from build123d import *

# Parameters (mm, degrees)
SKETCH_R        = 7.5
SKETCH_R_2      = 4.25
PAD_DEPTH       = 75
SKETCH001_W     = 19.415184
SKETCH001_H     = 42
POCKET_DEPTH    = 42
SKETCH002_R     = 11.25
POCKET001_DEPTH = 5
SKETCH003_R     = 1.75
HOLE_DEPTH      = 25
SKETCH004_R     = 1.5
HOLE001_DEPTH   = 25
HOLE001_TIPS_R  = 1.5
SKETCH005_R     = 11
POCKET002_DEPTH = 33
SKETCH006_R     = 11
POCKET003_DEPTH = 33


with BuildPart() as part:
    # Sketch → Pad (new body)
    with BuildSketch(Plane.XY):
        with BuildLine():
            ThreePointArc((-38.9, 12.5), (-51.4, 0), (-38.9, -12.5))
            Line((-38.9, -12.5), (30.9, -12.5))
            Line((95.9, -12.5), (30.9, -12.5))
            Line((95.9, -7.5), (95.9, -12.5))
            Line((34.678675, 11.915184), (95.9, -7.5))
            ThreePointArc((34.678675, 11.915184), (32.811831, 12.352931), (30.9, 12.5))
            Line((-38.9, 12.5), (30.9, 12.5))
        make_face()
        with Locations((-38.9, 0)):
            Circle(SKETCH_R, mode=Mode.SUBTRACT)
        with Locations((30.9, 0)):
            Circle(SKETCH_R_2, mode=Mode.SUBTRACT)
    extrude(amount=PAD_DEPTH)

    # Sketch001 (on Face3 of Pad) → Pocket (cut)
    with BuildSketch(Plane.YZ.offset(95.9)):
        with Locations((2.207592, 37.5)):
            Rectangle(SKETCH001_W, SKETCH001_H)
    extrude(amount=-POCKET_DEPTH, mode=Mode.SUBTRACT)

    # Sketch002 (on Face11 of Pocket) → Pocket001 (cut)
    with BuildSketch(Plane(origin=(0, -7.5, 0), x_dir=(-1, 0, 0), z_dir=(0, 1, 0))):
        with Locations((-74.9, 37.5)):
            Circle(SKETCH002_R)
    extrude(amount=-POCKET001_DEPTH, mode=Mode.SUBTRACT)

    # Sketch003 (on Face12 of Pocket001) → Hole (cut)
    with BuildSketch(Plane(origin=(0, -7.5, 0), x_dir=(-1, 0, 0), z_dir=(0, 1, 0))):
        with Locations((-90.4, 53)):
            Circle(SKETCH003_R)
        with Locations((-59.4, 53)):
            Circle(SKETCH003_R)
        with Locations((-59.4, 22)):
            Circle(SKETCH003_R)
        with Locations((-90.4, 22)):
            Circle(SKETCH003_R)
    extrude(amount=-HOLE_DEPTH, mode=Mode.SUBTRACT)

    # Sketch004 (on Face3 of Hole) → Hole001 (cut)
    with BuildSketch(Plane.XZ.offset(12.5)):
        with Locations((1.1, 72)):
            Circle(SKETCH004_R)
        with Locations((1.1, 54)):
            Circle(SKETCH004_R)
        with Locations((1.1, 21)):
            Circle(SKETCH004_R)
        with Locations((1.1, 3)):
            Circle(SKETCH004_R)
    extrude(amount=-HOLE001_DEPTH, mode=Mode.SUBTRACT)

    # Hole001 tips → Hole001 tip 1 section 0
    with BuildSketch(Plane.XZ.offset(-12.5), mode=Mode.PRIVATE) as hole001_tip_1_s0:
        with Locations((1.1, 72)):
            Circle(HOLE001_TIPS_R)
    loft([hole001_tip_1_s0.sketch, Vertex(1.1, 13.401291, 72)], mode=Mode.SUBTRACT)

    # Hole001 tips → Hole001 tip 2 section 0
    with BuildSketch(Plane.XZ.offset(-12.5), mode=Mode.PRIVATE) as hole001_tip_2_s0:
        with Locations((1.1, 54)):
            Circle(HOLE001_TIPS_R)
    loft([hole001_tip_2_s0.sketch, Vertex(1.1, 13.401291, 54)], mode=Mode.SUBTRACT)

    # Hole001 tips → Hole001 tip 3 section 0
    with BuildSketch(Plane.XZ.offset(-12.5), mode=Mode.PRIVATE) as hole001_tip_3_s0:
        with Locations((1.1, 21)):
            Circle(HOLE001_TIPS_R)
    loft([hole001_tip_3_s0.sketch, Vertex(1.1, 13.401291, 21)], mode=Mode.SUBTRACT)

    # Hole001 tips → Hole001 tip 4 section 0
    with BuildSketch(Plane.XZ.offset(-12.5), mode=Mode.PRIVATE) as hole001_tip_4_s0:
        with Locations((1.1, 3)):
            Circle(HOLE001_TIPS_R)
    loft([hole001_tip_4_s0.sketch, Vertex(1.1, 13.401291, 3)], mode=Mode.SUBTRACT)

    # Sketch005 (on Face5 of Hole001) → Pocket002 (cut)
    with BuildSketch(Plane.XY.offset(75)):
        with Locations((30.9, 0)):
            Circle(SKETCH005_R)
    extrude(amount=-POCKET002_DEPTH, mode=Mode.SUBTRACT)

    # Sketch006 (on Face4 of Pocket002) → Pocket003 (cut)
    with BuildSketch(Plane(origin=(0, 0, 0), x_dir=(1, 0, 0), z_dir=(0, 0, -1))):
        with Locations((30.9, 0)):
            Circle(SKETCH006_R)
    extrude(amount=-POCKET003_DEPTH, mode=Mode.SUBTRACT)


solid = part.part
The model under review builds one solid part; all positions refer to its coordinate system, in mm. A direction names the side the tool comes from. Round coordinates to 2 decimals unless told otherwise and drop trailing zeros. Loops run counter-clockwise (first coordinate to the right, second up) from the corner with the lowest first, then second, coordinate; pieces in that order, holes last. Notation, with made-up numbers: (75.25, 54) -> (85.25, 54) arc R4 cw to (85.25, 58) -> close; hole circle Ø7 at (-11.5, 48). An arc over 180 degrees is marked (long way). Return JSON: item names as keys, results as strings.
(1) For pin 1 (3 mm diameter, centred on x = 61.5, z = 60, fed in from +Y) (3 decimals); pin 2 (11 mm diameter, centred on x = 30.9, y = 0, fed in from -Z); pin 3 (2 mm diameter, centred on x = 59.5, z = 48.5, fed in from +Y), all flat-tipped, find the tip position at first contact; note any pin that passes through.
Solved:
{"pin 1": "y = 3.885", "pin 2": "z = 33", "pin 3": "y = -7.5"}
(2) For faces 4 (the flat face through (66, -7.5, 47)), 5 (the cylindrical face through (35.976, -9.759, 58.731)), 6 (the flat face through (31, 5, 33)), 7 (the flat face through (51.256, 6.658, 36.975)), list the 3-axis set-ups (+Z, -Z, +X, -X, +Y, -Y) from which the entire face can be reached by the end or side of a thin tool; tool diameter is ignored.
Solved:
{"face 4": "+X, +Y", "face 5": "+Z", "face 6": "-Z", "face 7": "+Z, -Z, +X, +Y"}
(3) Add section B-B on y = 0. Write out the cut boundary in (x, z), plus the area to 3 significant figures.
Solved:
{"outline": "(-51.4, 0) -> (-46.4, 0) -> (-46.4, 75) -> (-51.4, 75) -> close; (-31.4, 0) -> (19.9, 0) -> (19.9, 33) -> (26.65, 33) -> (26.65, 42) -> (19.9, 42) -> (19.9, 75) -> (-31.4, 75) -> close; (35.15, 33) -> (41.9, 33) -> (41.9, 0) -> (72.25, 0) -> (72.25, 16.5) -> (53.9, 16.5) -> (53.9, 58.5) -> (72.25, 58.5) -> (72.25, 75) -> (41.9, 75) -> (41.9, 42) -> (35.15, 42) -> close; hole circle Ø3 at (1.1, 3); hole circle Ø3 at (1.1, 21); hole circle Ø3 at (1.1, 54); hole circle Ø3 at (1.1, 72)", "area": "5,820 mm2"}
(4) For line 1 (Z direction, x = 90.4, y = -10.1); line 2 (Y direction, x = 30.9, z = 68.5); line 3 (Z direction, x = 1.1, y = -5.5), list the stretches that pass through material, from the lowest coordinate up.
Solved:
{"line 1": "0 to 20.25, 23.75 to 51.25, 54.75 to 75", "line 2": "-12.5 to -11, 11 to 12.5", "line 3": "0 to 1.5, 4.5 to 19.5, 22.5 to 52.5, 55.5 to 70.5, 73.5 to 75"}
(5) Add section C-C on x = 79. Write out the cut boundary in (y, z).
Solved:
{"outline": "(-12.5, 0) -> (-2.14, 0) -> (-2.14, 16.5) -> (-7.5, 16.5) -> (-7.5, 27.02) -> (-12.5, 27.02) -> close; (-12.5, 47.98) -> (-7.5, 47.98) -> (-7.5, 58.5) -> (-2.14, 58.5) -> (-2.14, 75) -> (-12.5, 75) -> close"}
(6) Add section A-A on z = 3. Write out the cut boundary in (x, y).
Solved:
{"outline": "(-38.9, -12.5) -> (-0.4, -12.5) -> (-0.4, 12.5) -> (-38.9, 12.5) arc R12.5 ccw to start; (2.6, -12.5) -> (95.9, -12.5) -> (95.9, -7.5) -> (34.68, 11.92) arc R12.5 ccw to (30.9, 12.5) -> (2.6, 12.5) -> close; hole circle Ø15 at (-38.9, 0); hole circle Ø22 at (30.9, 0)"}
(7) Add section D-D on z = 46.5. Write out the cut boundary in (x, y).
Solved:
{"outline": "(-38.9, -12.5) -> (68.15, -12.5) -> (68.15, -7.5) -> (53.9, -7.5) -> (53.9, 5.82) -> (34.68, 11.92) arc R12.5 ccw to (30.9, 12.5) -> (-38.9, 12.5) arc R12.5 ccw to start; (81.65, -12.5) -> (95.9, -12.5) -> (95.9, -7.5) -> (81.65, -7.5) -> close; hole circle Ø15 at (-38.9, 0); hole circle Ø22 at (30.9, 0)"}
(8) The part is to be moulded in two halves that separate along Y. For faces 1 (the flat face through (28, -12.5, 37)), 2 (the cylindrical face through (0.905, -0.175, 22.487)), 3 (the cylindrical face through (-46.393, 0.33, 36.975)), say which applies: released by +Y, released by -Y, zero draft, split by the parting line, or undercut.
Solved:
{"face 1": "released by -Y", "face 2": "zero draft", "face 3": "undercut"}
